Could you check a few things on this drawing? It's one solid part, dimensions in mm from its lowest x, y, z. A direction names the side the tool comes from. Coordinates: 2 decimals unless noted, no trailing zeros. Order: outer loops, then holes, each group sorted by start corner. A loop starts at its lowest first (then second) coordinate and runs counter-clockwise, first axis right, second up. Notation, with made-up numbers: M 84.25,-34 L 100.25,-34 A35 cw 100.25,-1 Z; hole C 85.5,52 d1. An arc over 180 degrees is marked long. Write item = value, one per line. Start each with the question number.
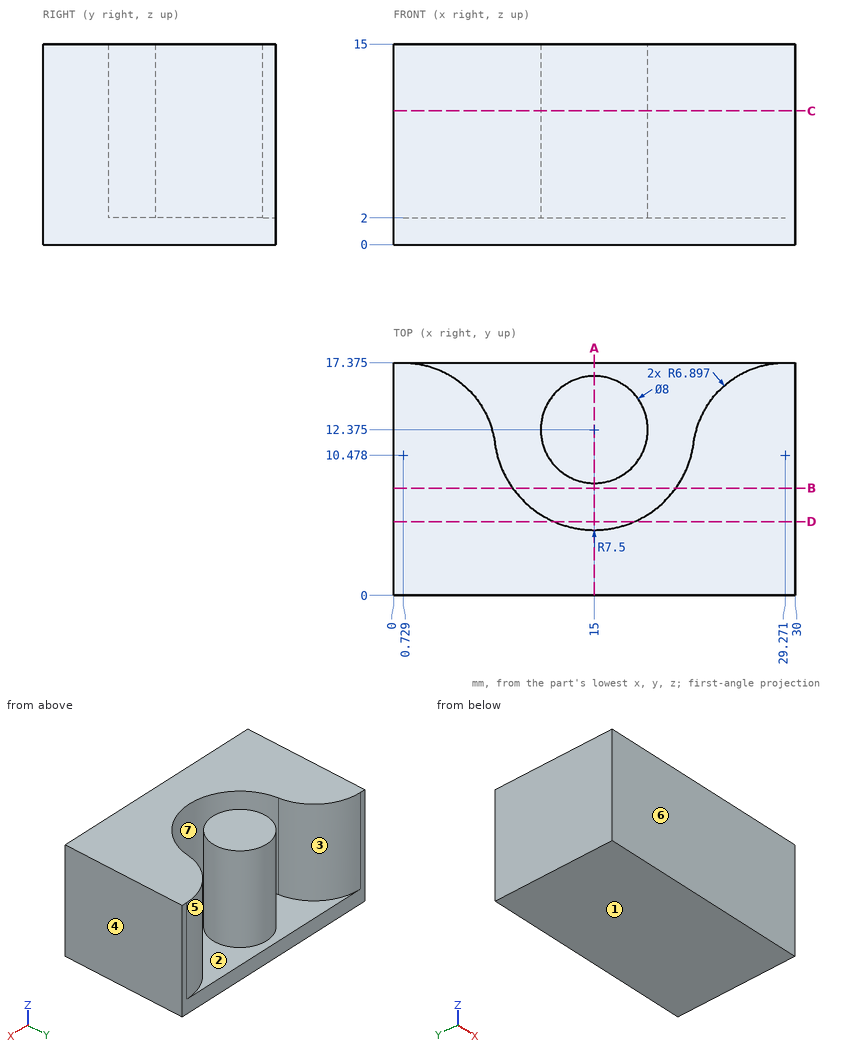
(1) Imagine slicing it at C-C on z = 10. List the corners of the cut face in (x, y) for me (1 decimal), plus the area to 3 significant figures.
(2) Please list where these lines run through material, in increasing order: probe 1 along X at (y, z) = (15, 8.75) (1 decimal); probe 2 along X at (y, z) = (14, 6) (1 decimal); probe 3 along X at (y, z) = (16.5, 11.5). Write a range as from..to.
(3) Imagine slicing it at A-A on x = 15. List the corners of the cut face in (y, z) for me (1 decimal).
(4) Imagine slicing it at B-B on y = 8. List the corners of the cut face in (x, z) for me.
(5) Imagine slicing it at D-D on y = 5.5. List the corners of the cut face in (x, z) for me.
(6) Thinking about a two-plate mould opening in Y: for the marked faces 4, 5, 6 and 7, which applies, released by +Y, released by -Y, zero draft, split by the parting line, or undercut?
(7) For the marked faces 1, 2 and 3, which set-ups out of +Z, -Z, +X, -X, +Y, -Y let a thin tool reach every point of the face, with its end or its side?
(8) Will this pin go through, and if not, where does the flat tip stop? P1, Ø1.5, axis at x = 25.5, z = 3, coming from the +Y side.
Response:
q1.outline = M 0,0 L 30,0 L 30,17.4 L 29.3,17.4 A6.9 ccw 22.4,11.4 A7.5 cw 7.6,11.4 A6.9 ccw 0.7,17.4 L 0,17.4 Z; C 15,12.4 d8
q1.area = 389 mm2
q2.probe_1 = 0..5.9, 12..18, 24.1..30
q2.probe_2 = 0..6.7, 11.3..18.7, 23.3..30
q2.probe_3 = 0..4.09, 25.91..30
q3.outline = M 0,0 L 17.4,0 L 17.4,2 L 16.4,2 L 16.4,15 L 8.4,15 L 8.4,2 L 4.9,2 L 4.9,15 L 0,15 Z
q4.outline = M 0,0 L 30,0 L 30,15 L 21.09,15 L 21.09,2 L 8.91,2 L 8.91,15 L 0,15 Z
q5.outline = M 0,0 L 30,0 L 30,15 L 18,15 L 18,2 L 12,2 L 12,15 L 0,15 Z
q6.face_4 = zero draft
q6.face_5 = released by +Y
q6.face_6 = released by -Y
q6.face_7 = undercut
q7.face_1 = -Z, +X, -X, +Y, -Y
q7.face_2 = +Z
q7.face_3 = +Z, +Y
q8.P1 = 16.68
